Autodesk Inventor part; units mm, degrees
ref_plane "YZ Plane" through (0, 0, 0) normal (1, 0, 0) x (0, 1, 0)
ref_plane "XZ Plane" through (0, 0, 0) normal (0, 1, 0) x (-1, 0, 0)
ref_plane "XY Plane" through (0, 0, 0) normal (0, 0, 1) x (1, 0, 0)
sketch "スケッチ1" plane through (0, 0, 0) normal (0, 0, 1) x (1, 0, 0)
  line L0 (-4.25, 5) -> (0, 5)
  line L1 (4.25, 5) -> (4.25, 0)
  line L2 (4.25, 0) -> (-4.25, 0)
  line L3 (-4.25, 0) -> (-4.25, 5)
  line L4 (-2.5, 0) -> (0, 0)
  line L5 (2.5, 0) -> (2.5, -8)
  line L6 (2.5, -8) -> (0, -8)
  line L7 (-2.5, -8) -> (-2.5, 0)
  line L8 (0, 5) -> (0, -8)
  line L9 (0, 5) -> (4.25, 5)
  line L10 (0, 0) -> (2.5, 0)
  line L11 (0, -8) -> (-2.5, -8)
  point P0 (0, 0)
  dimension "d0" = 5
  dimension "d1" = 2.5
  dimension "d2" = 8
  dimension "d3" = 8.5
  dimension "d4" = 4.25
  dimension "d5" = 5
  dimension "d18" = 5
revolve "回転1" add sketch "スケッチ1" angle 360 about axis through (0, 5, 0) along (0, -1, 0) contours L0 L8 L2 L3 | L8 L11 L7 L2
sketch "スケッチ2" plane through (0, 5, 0) normal (0, 1, 0) x (1, 0, 0)
  line L0 (0, 2.3094) -> (2, 1.1547)
  line L1 (2, 1.1547) -> (2, -1.1547)
  line L2 (2, -1.1547) -> (0, -2.3094)
  line L3 (0, -2.3094) -> (-2, -1.1547)
  line L4 (-2, -1.1547) -> (-2, 1.1547)
  line L5 (-2, 1.1547) -> (0, 2.3094)
  point P0 (0, 0)
  dimension "d9" = 4
extrude "押し出し1" cut sketch "スケッチ2" against normal blind 3
chamfer "面取り1" distance 0.1 angle 45 2 edges at (4.25, 5, 0) (4.25, 0, 0)
chamfer "面取り2" distance 0.2 angle 45 6 edges at (1, 5, 1.7321) (-1, 5, 1.7321) (-2, 5, 0) (-1, 5, -1.7321) (1, 5, -1.7321) (2, 5, 0)
thread "ねじ2"
equation "\"d18\" = d0"
properties part number "M5_8mm"
CAD build for the part. Positions are in the model's coordinates, mm. A direction names the side the tool comes from. Coordinates: 2 decimals unless noted, no trailing zeros. Order: outer loops, then holes, each group sorted by start corner. A loop starts at its lowest first (then second) coordinate and runs counter-clockwise, first axis right, second up. Notation, with made-up numbers: (65, 50) -> (104, 50) arc R28 ccw to (104, 73) -> close; hole circle Ø5 at (-31, 49). An arc over 180 degrees is marked (long way). Use one line per item in the form item = value. Start each with the question number.
1) Tool access for faces 1 (the flat face through (-1.014, 3.42, -1.724)), 2 (the flat face through (-2, 0, 2)), 3 (the flat face through (-2, 5, 2)): list every direction of +Z, -Z, +X, -X, +Y, -Y with a clear straight run to the whole face (end or side of a thin tool).
2) Drop flat-ended pins along their axis: pin 1 (1.5 mm diameter, centred on y = -3, z = -1.5, fed in from -X); pin 2 (1.2 mm diameter, centred on y = 3, z = -0.5, fed in from -X). Give the stop position or say it passes through.
3) Band-saw the part on B-B on z = 0. Give the cut face in (x, y), then the cut area to 3 significant figures.
4) Drill centre lines: L1, parallel to Y at x = 0.5, z = -2.75; L2, parallel to Y at x = -0.25, z = 0.25; L3, parallel to Z at x = -1, y = 2.5. Where is each one in solid material? Low to high. Write a range as [from, to].
5) Pull direction Z, two halves, no side cores. Call faces 4 (the flat face through (1.014, 3.42, 1.724)), 5 (the cylindrical face through (-2.285, 2.534, 3.584)), 6 (the flat face through (0, -8, 0)): +Z half, -Z half, draft (parallel to the pull), parting line (faces both ways), or undercut.
6) Band-saw the part on C-C on y = 0.25. Give the cut face in (x, z).
7) Band-saw the part on A-A on y = 2.25. Give the cut face in (x, z).
8) Band-saw the part on D-D on y = -3. Give the cut face in (x, z).
Entries:
q1.face_1 = +Y
q1.face_2 = -Y
q1.face_3 = +Z, -Z, +X, -X, +Y
q2.pin_1 = -2.38
q2.pin_2 = -4.25
q3.outline = (-4.25, 0.1) -> (-4.15, 0) -> (-2.5, 0) -> (-2.5, -8) -> (2.5, -8) -> (2.5, 0) -> (4.15, 0) -> (4.25, 0.1) -> (4.25, 4.9) -> (4.15, 5) -> (2.2, 5) -> (2, 4.8) -> (2, 2) -> (-2, 2) -> (-2, 4.8) -> (-2.2, 5) -> (-4.15, 5) -> (-4.25, 4.9) -> close
q3.area = 70.4 mm2
q4.L1 = [0, 5]
q4.L2 = [-8, 2]
q4.L3 = [-4.13, -1.73], [1.73, 4.13]
q5.face_4 = undercut
q5.face_5 = parting line
q5.face_6 = draft
q6.outline = circle Ø8.5 at (0, 0)
q7.outline = circle Ø8.5 at (0, 0); hole (-2, -1.15) -> (0, -2.31) -> (2, -1.15) -> (2, 1.15) -> (0, 2.31) -> (-2, 1.15) -> close
q8.outline = circle Ø5 at (0, 0)
